Part model, mm, in its own coordinate system. A direction names the side the tool comes from. Give positions to 0.01 mm unless a question says otherwise; leave off trailing zeros. Loops run counter-clockwise (first coordinate to the right, second up) from the corner with the lowest first, then second, coordinate; pieces in that order, holes last. Notation, with made-up numbers: M 39.5,71 L 76.5,71 A27 ccw 76.5,92 Z; hole C -37.75,78.25 d7. An arc over 180 degrees is marked long. Answer in a Markdown table with one row per item.
from build123d import *

# Parameters (mm, degrees)
BOSS_EXTRUDE1_DEPTH = 15
FILLET2_R           = 5
FILLET3_R           = 5
FILLET4_R           = 5
CHAMFER1_SIZE       = 2
BOSS_EXTRUDE2_DEPTH = 7.5
FILLET5_R           = 3
FILLET6_R           = 3.5
FILLET7_R           = 3.5
FILLET8_R           = 1.5
FILLET9_R           = 2


with BuildPart() as part:
    # Sketch1 → Boss-Extrude1 (new, symmetric)
    with BuildSketch(Plane(origin=(0, 0, 0), x_dir=(0, 0, -1), z_dir=(1, 0, 0))):
        Polygon((0, 0), (-15, 0), (-69.940788655, 0), (-69.940788655, -3.95), (-49.940788655, -3.95), (-49.940788655, -3.7), (-17.940788655, -3.7), (-17.940788655, -3.95), (-13.226857143, -3.95), (-6, -3.95), (-6, -56), (46, -56), (46, -34), (40, -34), (40, -50), (0, -50), align=None)
    extrude(amount=BOSS_EXTRUDE1_DEPTH, both=True)

    # Fillet2
    fillet2_edges = [part.edges().sort_by_distance(p)[0] for p in [
        (0, 0, 0),
    ]]
    fillet(fillet2_edges, radius=FILLET2_R)

    # Fillet3
    fillet3_edges = [part.edges().sort_by_distance(p)[0] for p in [
        (0, -50, 0),
        (0, -50, -40),
    ]]
    fillet(fillet3_edges, radius=FILLET3_R)

    # Fillet4
    fillet4_edges = [part.edges().sort_by_distance(p)[0] for p in [
        (0, -56, -46),
        (0, -56, 6),
    ]]
    fillet(fillet4_edges, radius=FILLET4_R)

    # Chamfer1
    # the kernel refuses this chamfer: 2 mm, written as the material it takes off along each edge
    with BuildSketch(Plane(origin=(-20.143365976, -3.95, 69.940788655), x_dir=(0, -0.027495876610586414, -0.9996219169112968), z_dir=(1, 0, 0))) as chamfer1_piece_1:
        Polygon((CHAMFER1_SIZE * 0.999621916911, CHAMFER1_SIZE * 0.0274958766106), (-CHAMFER1_SIZE * 0.0274958766106, CHAMFER1_SIZE * 0.999621916911), (0, 0), align=None)
    extrude(amount=40.286731952, mode=Mode.SUBTRACT)
    with BuildSketch(Plane(origin=(-20.143365976, 0, 69.940788655), x_dir=(0, 0.027495876610585952, -0.9996219169112968), z_dir=(1, 0, 0))) as chamfer1_piece_2:
        Polygon((CHAMFER1_SIZE * 0.999621916911, -CHAMFER1_SIZE * 0.0274958766106), (-CHAMFER1_SIZE * 0.0274958766106, -CHAMFER1_SIZE * 0.999621916911), (0, 0), align=None)
    extrude(amount=40.286731952, mode=Mode.SUBTRACT)

    # Sketch3 → Boss-Extrude2 (add, symmetric)
    with BuildSketch(Plane(origin=(0, 0, 0), x_dir=(0, 0, -1), z_dir=(1, 0, 0))):
        Polygon((19, -56), (19, -74), (35, -74), (35, -64), (31, -64), (31, -70), (23, -70), (23, -56), align=None)
    extrude(amount=BOSS_EXTRUDE2_DEPTH, both=True)

    # Fillet5
    fillet5_edges = [part.edges().sort_by_distance(p)[0] for p in [
        (0, -56, -23),
        (0, -56, -19),
    ]]
    fillet(fillet5_edges, radius=FILLET5_R)

    # Fillet6
    fillet6_edges = [part.edges().sort_by_distance(p)[0] for p in [
        (0, -70, -31),
        (0, -70, -23),
    ]]
    fillet(fillet6_edges, radius=FILLET6_R)

    # Fillet7
    fillet7_edges = [part.edges().sort_by_distance(p)[0] for p in [
        (0, -74, -19),
        (0, -74, -35),
    ]]
    fillet(fillet7_edges, radius=FILLET7_R)

    # Fillet8
    fillet8_edges = [part.edges().sort_by_distance(p)[0] for p in [
        (0, -64, -35),
        (0, -64, -31),
    ]]
    fillet(fillet8_edges, radius=FILLET8_R)

    # Fillet9
    fillet9_edges = [part.edges().sort_by_distance(p)[0] for p in [
        (0, -34, -40),
        (0, -34, -46),
    ]]
    fillet(fillet9_edges, radius=FILLET9_R)


solid = part.part
(1) Pull direction Y, two halves, no side cores. Call faces 6 (the face through (0, -44, -46)), 7 (the face through (0, -55, 4)), 8 (the face through (-0.11, -56.86, -23.9)): +Y half, -Y half, draft (parallel to the pull), parting line (faces both ways), or undercut.
Recorded:
| item | result |
|---|---|
| face 6 | draft |
| face 7 | -Y half |
| face 8 | undercut |
(2) Saw through at B-B (x = -10.25). Write the cut outline in (y, z) (3 decimals), plus the area to 3 significant figures.
Recorded:
| item | result |
|---|---|
| outline | M -56,-41 A5 ccw -51,-46 L -36,-46 A2 ccw -34,-44 L -34,-42 A2 ccw -36,-40 L -45,-40 A5 cw -50,-35 L -50,-5 A5 cw -45,0 L -5,0 A5 ccw 0,5 L 0,67.941 L -1.975,69.916 L -3.95,67.941 L -3.95,49.941 L -3.7,49.941 L -3.7,17.941 L -3.95,17.941 L -3.95,6 L -51,6 A5 ccw -56,1 Z |
| area | 941 mm^2 |
(3) Which spindle directions (+Z, -Z, +X, -X, +Y, -Y) get a long thin tool onto all of the face, cutting with end or side? Do faces 1 (the face through (-0.11, -68.95, -24)), 2 (the face through (0, -68, -35)), 3 (the face through (0, -25, 0)), 4 (the face through (0, -3.95, 12)), 5 (the face through (7.5, -69, -23)). Say none if no direction does.
Recorded:
| item | result |
|---|---|
| face 1 | +X, -X |
| face 2 | -Z, +X, -X, -Y |
| face 3 | +X, -X, +Y |
| face 4 | +Z, +X, -X, -Y |
| face 5 | +Z, -Z, +X, -Y |
(4) Drill centre lines: line 1 along Z through (x, y) = (-11.75, -10.5); line 2 along Y through (x, z) = (-1.25, 54); line 3 along Z through (x, y) = (0, -59.5). Where is each one in solid material? Low to high.
Recorded:
| item | result |
|---|---|
| line 1 | z = 0 to 6 |
| line 2 | y = -3.95 to 0 |
| line 3 | z = -23 to -19 |
(5) Saw through at A-A (y = -48). Write the cut outline in (x, z), plus the area to 3 significant figures.
Recorded:
| item | result |
|---|---|
| outline | M -15,-46 L 15,-46 L 15,-39 L -15,-39 Z; M -15,-1 L 15,-1 L 15,6 L -15,6 Z |
| area | 420 mm^2 |
(6) Saw through at C-C (z = -11.5). Write the cut outline in (x, y), plus the area to 3 significant figures.
Recorded:
| item | result |
|---|---|
| outline | M -15,-56 L 15,-56 L 15,-50 L -15,-50 Z |
| area | 180 mm^2 |
(7) Saw through at D-D (y = -29.5). Write the cut outline in (x, z), plus the area to 3 significant figures.
Recorded:
| item | result |
|---|---|
| outline | M -15,0 L 15,0 L 15,6 L -15,6 Z |
| area | 180 mm^2 |
(8) Pin check, flat tips, straight feed: pin 1 Ø1.5 at (x, z) = (9, -22.5) entering from -Y; pin 2 Ø6 at (x, z) = (2, 14) entering from -Y; pin 3 Ø3 at (x, y) = (10.5, -48) entering from +Z; pin 4 Ø12 at (y, z) = (-17, 17.5) entering from -X. Stop position of each tip, or through.
Recorded:
| item | result |
|---|---|
| pin 1 | stops at y = -56 |
| pin 2 | stops at y = -3.95 |
| pin 3 | stops at z = 6 |
| pin 4 | passes through |
